```python
from build123d import *

# Parameters (mm, degrees)
BOSS_EXTRUDE1_DEPTH    = 52
SKETCH3_R              = 5
CUT_EXTRUDE2_DEPTH     = 78.803153053
M2_5_CLEARANCE_HOLE1_D = 2.9
M4_CLEARANCE_HOLE1_D   = 4.5


with BuildPart() as part:
    # Sketch1 → Boss-Extrude1 (new body)
    with BuildSketch(Plane.XY):
        Polygon((0, 0), (0, 36.825), (3.175, 36.825), (3.175, -3.175), (-41.825, -3.175), (-41.825, 0), align=None)
    extrude(amount=BOSS_EXTRUDE1_DEPTH)

    # Sketch3 → Cut-Extrude2 (cut, through all)
    with BuildSketch(Plane(origin=(0, -3.175, 0), x_dir=(-1, 0, 0), z_dir=(0, -1, 0))):
        with Locations(Location((22.825, -38.5, 0), (0, 0, 180))):
            Circle(SKETCH3_R)
    extrude(amount=-CUT_EXTRUDE2_DEPTH, mode=Mode.SUBTRACT)

    # M2.5 Clearance Hole1 (through all)
    with Locations(Plane(origin=(0, -3.175, 0), x_dir=(-1, 0, 0), z_dir=(0, -1, 0))):
        with Locations((7.825, -9), (37.825, -9), (7.825, -26), (37.825, -26), (37.825, -43), (7.825, -43)):
            Hole(M2_5_CLEARANCE_HOLE1_D / 2)

    # M4 Clearance Hole1 (through all)
    with Locations(Plane(origin=(3.175, 0, 0), x_dir=(0, 0, -1), z_dir=(1, 0, 0))):
        with Locations((-26, 28.138708499), (-18, 24.825), (-14.686291501, 16.825), (-18, 8.825), (-26, 5.511291501), (-34, 8.825), (-37.313708499, 16.825), (-34, 24.825)):
            Hole(M4_CLEARANCE_HOLE1_D / 2)


solid = part.part
```
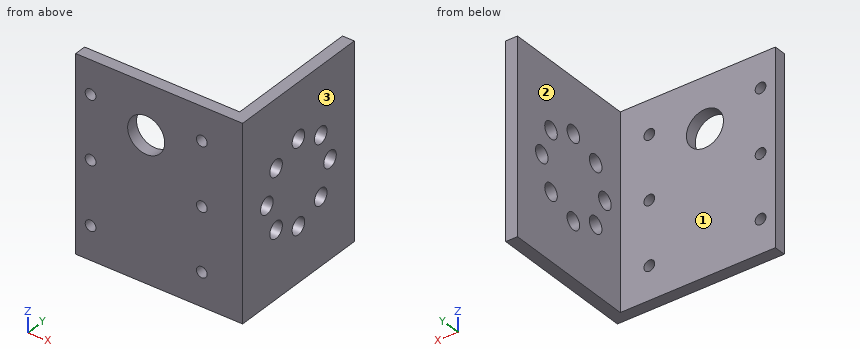
Work out the finished part from the listing and answer in its coordinate system (mm). Face numbers are marked on the shaded views. Round coordinates to 2 decimals unless told otherwise and drop trailing zeros. Loops run counter-clockwise (first coordinate to the right, second up) from the corner with the lowest first, then second, coordinate; pieces in that order, holes last.
(1) The part is cut by section A-A, the plane z = 9. Give the vertices of the cut face in (x, y) (3 decimals).
Computed values:
outline: (-41.825, -3.175) - (-39.275, -3.175) - (-39.275, 0) - (-41.825, 0) - close; (-36.375, -3.175) - (-9.275, -3.175) - (-9.275, 0) - (-36.375, 0) - close; (-6.375, -3.175) - (3.175, -3.175) - (3.175, 36.825) - (0, 36.825) - (0, 0) - (-6.375, 0) - close
(2) The mould has two halves that part along X. Classify the marked faces 1, 2 and 3: pulls with the +X half, pulls with the -X half, needs draft (parallel to the pull), parting line crosses it, or undercut.
Computed values:
face 1: needs draft
face 2: pulls with the -X half
face 3: pulls with the +X half
(3) The part is cut by section D-D, the plane z = 38.5. Give the vertices of the cut face in (x, y) (3 decimals), and give its area (3 significant figures).
Computed values:
outline: (-41.825, -3.175) - (-27.825, -3.175) - (-27.825, 0) - (-41.825, 0) - close; (-17.825, -3.175) - (3.175, -3.175) - (3.175, 14.913) - (0, 14.913) - (0, 0) - (-17.825, 0) - close; (0, 18.737) - (3.175, 18.737) - (3.175, 36.825) - (0, 36.825) - close
area: 216 mm2
(4) Find the intervals of material crossed by L1, parallel to X at y = -2.15, z = 26 (3 decimals); L2, parallel to Y at x = 1.35, z = 18 (3 decimals); L3, parallel to X at y = -0.75, z = 43 (3 decimals), in increasing order.
Computed values:
L1: x = -41.825 to -39.275, -36.375 to -9.275, -6.375 to 3.175
L2: y = -3.175 to 6.575, 11.075 to 22.575, 27.075 to 36.825
L3: x = -41.825 to -39.275, -36.375 to -25.004, -20.646 to -9.275, -6.375 to 3.175
(5) The part is cut by section C-C, the plane z = 26. Give the vertices of the cut face in (x, y) (3 decimals), and give its area (3 significant figures).
Computed values:
outline: (-41.825, -3.175) - (-39.275, -3.175) - (-39.275, 0) - (-41.825, 0) - close; (-36.375, -3.175) - (-9.275, -3.175) - (-9.275, 0) - (-36.375, 0) - close; (-6.375, -3.175) - (3.175, -3.175) - (3.175, 3.261) - (0, 3.261) - (0, 0) - (-6.375, 0) - close; (0, 7.761) - (3.175, 7.761) - (3.175, 25.889) - (0, 25.889) - close; (0, 30.389) - (3.175, 30.389) - (3.175, 36.825) - (0, 36.825) - close
area: 213 mm2
(6) Each of these flat-tipped pins is pushed along its axis until it touches: P1, Ø4, axis at x = -7.825, z = 26, coming from the +Y side; P2, Ø9, axis at x = -22.825, z = 38.5, coming from the -Y side. Where does it stop, or does it pass through?
Computed values:
P1: stops at y = 0
P2: passes through
(7) The part is cut by section B-B, the plane x = -20. Give the vertices of the cut face in (y, z) (3 decimals), and give its area (3 significant figures).
Computed values:
outline: (-3.175, 0) - (0, 0) - (0, 34.375) - (-3.175, 34.375) - close; (-3.175, 42.625) - (0, 42.625) - (0, 52) - (-3.175, 52) - close
area: 139 mm2
